```python
from build123d import *

# Parameters (mm, degrees)
F0_R     = 14.2875
F0_W     = 82.55
F0_H     = 368.3
F1_DEPTH = 4.7625


# Not quite as in the source:
# - a feature names something its author has since deleted; it is built from what else it names


with BuildPart() as f1:
    # F0 (on Top) → F1 (new body)
    with BuildSketch(Plane.XY):
        Polygon((19.05, -114.3), (-101.6, -114.3), (-101.6, -254), (101.6, -254), (101.6, -114.3), align=None)
        with Locations((-79.375, -156.21)):
            Circle(F0_R, mode=Mode.SUBTRACT)
        with Locations((47.625, -156.21)):
            Circle(F0_R, mode=Mode.SUBTRACT)
        Polygon((202.565, 254), (101.6, 254), (101.6, -114.3), (101.6, -254), (202.565, -254), align=None)
        with Locations((60.325, 69.85)):
            Rectangle(F0_W, F0_H)
        with Locations((47.625, 229.87)):
            Circle(F0_R, mode=Mode.SUBTRACT)
    extrude(amount=F1_DEPTH)


solid = f1.part
```
Work out the finished part from the listing and answer in its coordinate system (mm). Round coordinates to 2 decimals unless told otherwise and drop trailing zeros. Loops run counter-clockwise (first coordinate to the right, second up) from the corner with the lowest first, then second, coordinate; pieces in that order, holes last.
(1) Each of these flat-tipped pins is pushed along its axis until it touches: P1, Ø2.5, axis at y = 158.5, z = 2.5, coming from the -X side; P2, Ø1.5, axis at x = -33.5, z = 2, coming from the +Y side; P3, Ø17, axis at x = 47.625, y = 229.87, coming from the -Z side. Where does it stop, or does it pass through?
Computed values:
P1: stops at x = 19.05
P2: stops at y = -114.3
P3: passes through
(2) The part is cut by section B-B, the plane y = -156.21. Give the vertices of the cut face in (x, z) (1 decimal), and give its area (3 significant figures).
Computed values:
outline: (-101.6, 0) - (-93.7, 0) - (-93.7, 4.8) - (-101.6, 4.8) - close; (-65.1, 0) - (33.3, 0) - (33.3, 4.8) - (-65.1, 4.8) - close; (61.9, 0) - (202.6, 0) - (202.6, 4.8) - (61.9, 4.8) - close
area: 1,180 mm2
(3) The part is cut by section A-A, the plane z = 2.2. Give the number of separate pieces and of enclosed holes in the cut face, and give its area (3 significant figures).
Computed values:
separate pieces: 1
enclosed holes: 3
area: 108,000 mm2
(4) The mould has two halves that part along Y. Classify faces 1 (the flat face through (82, -53, 0)), 2 (the cylindrical face through (44.53, -170.16, 2.35)): pulls with the +Y half, pulls with the -Y half, needs draft (parallel to the pull), parting line crosses it, or undercut.
Computed values:
face 1: needs draft
face 2: undercut
(5) The part is cut by section D-D, the plane x = -73. Give the vertices of the cut face in (y, z), and give its area (3 significant figures).
Computed values:
outline: (-254, 0) - (-169, 0) - (-169, 4.76) - (-254, 4.76) - close; (-143.42, 0) - (-114.3, 0) - (-114.3, 4.76) - (-143.42, 4.76) - close
area: 544 mm2
(6) Find the intervals of material crossed by L1, parallel to Y at x = 48.5, z = 4.3; L2, parallel to X at y = -148.5, z = 3.8 (3 decimals); L3, parallel to X at y = -151, z = 1 (3 decimals), in increasing order.
Computed values:
L1: y = -254 to -170.47, -141.95 to 215.61, 244.13 to 254
L2: x = -101.6 to -91.404, -67.346 to 35.596, 59.654 to 202.565
L3: x = -101.6 to -92.679, -66.071 to 34.321, 60.929 to 202.565
